```python
from build123d import *


with BuildPart() as part:
    # Croquis1 → Revolución1 (revolve)
    with BuildSketch(Plane.XY):
        with BuildLine():
            Line((0.6, 25), (3.542, 25))
            ThreePointArc((3.542, 25), (3.966264069, 25.175735931), (4.142, 25.6))
            Line((4.142, 25.6), (4.142, 27.857333437))
            ThreePointArc((4.142, 27.857333437), (3.428, 30), (4.142, 32.142666563))
            Line((4.142, 32.142666563), (4.142, 35))
            Line((4.142, 35), (0.6, 35))
            ThreePointArc((0.6, 35), (0.175735931, 34.824264069), (0, 34.4))
            Line((0, 34.4), (0, 25.6))
            ThreePointArc((0, 25.6), (0.175735931, 25.175735931), (0.6, 25))
        make_face()
    revolve(axis=Axis((3.542, 0, 0), (-1, 0, 0)))


solid = part.part
```
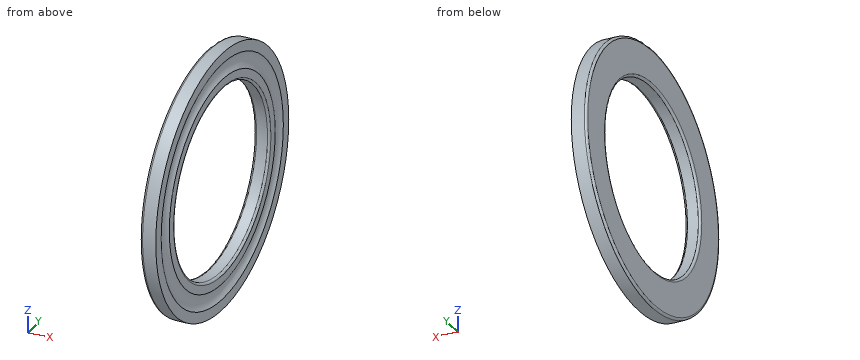
The model under review builds one solid part; all positions refer to its coordinate system, in mm. Round coordinates to 2 decimals unless told otherwise and drop trailing zeros. Write each loop counter-clockwise with the first axis right and the second up, starting at its lowest first coordinate (ties: lowest second). Pieces come first, ordered by that corner, then holes.
(1) Wall thickness on L1, parallel to Y at x = 2.3, z = 0; L2, parallel to Z at x = 3.9, y = -4: over which ranges is each line inside the solid? List them lowest first.
(2) Insertion check: pin 1 (1.5 mm diameter, centred on x = 2, z = 19, fed in from -Y); pin 2 (1 mm diameter, centred on x = 3, y = 5.5, fed in from +Z); pin 3 (4 mm diameter, centred on y = 23, z = 4, fed in from -X). Each pin has a flat end and moves straight along its axis. Give the tip position at first contact, or say it passes through.
(3) We need section C-C on x = 2.25. Give the boundary of the cut face in (y, z).
(4) We need section A-A on z = 0. Give the boundary of the cut face in (x, y), and give its area (3 significant figures).
Findings below:
1. L1: y = -35 to -25, 25 to 35
1. L2: z = -34.77 to -31.52, -27.94 to -24.8, 24.8 to 27.94, 31.52 to 34.77
2. pin 1: stops at y = -29.87
2. pin 2: stops at z = 34.64
2. pin 3: stops at x = 0.06
3. outline: circle Ø70 at (0, 0); hole circle Ø50 at (0, 0)
4. outline: (0, -34.4) arc R0.6 ccw to (0.6, -35) - (4.14, -35) - (4.14, -32.14) arc R3.57 cw to (4.14, -27.86) - (4.14, -25.6) arc R0.6 ccw to (3.54, -25) - (0.6, -25) arc R0.6 ccw to (0, -25.6) - close; (0, 25.6) arc R0.6 ccw to (0.6, 25) - (3.54, 25) arc R0.6 ccw to (4.14, 25.6) - (4.14, 27.86) arc R3.57 cw to (4.14, 32.14) - (4.14, 35) - (0.6, 35) arc R0.6 ccw to (0, 34.4) - close
4. area: 78.2 mm2
